The figure shows three views and two pictorial views of one solid part (mm, origin at its lowest corner). Answer the questions. A direction names the side the tool comes from. Coordinates: 2 decimals unless noted, no trailing zeros. Loops run counter-clockwise (first coordinate to the right, second up) from the corner with the lowest first, then second, coordinate; pieces in that order, holes last.
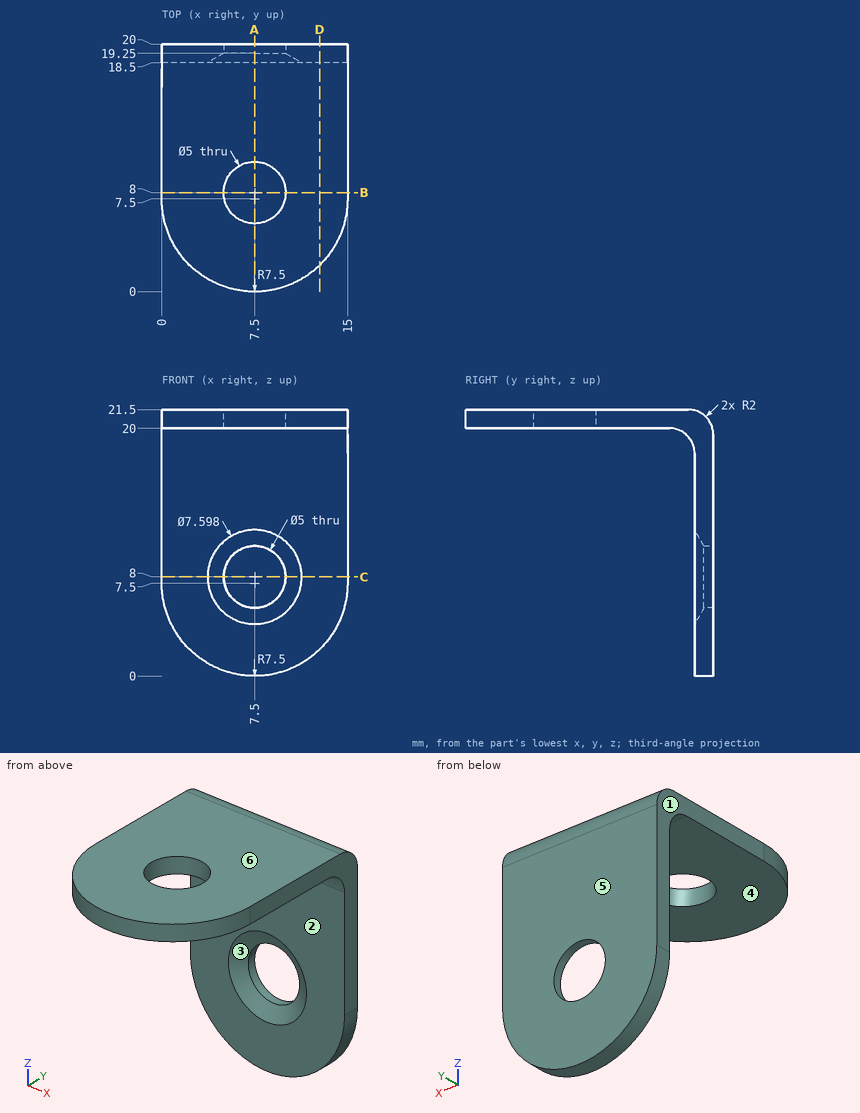
1. Straight lines are drawn through the part: probe 1 along X at (y, z) = (8, 21); probe 2 along Z at (x, y) = (13.5, 15.75); probe 3 along Y at (x, z) = (9, 18). For each, find the intervals that lie inside material, in ascending order.
2. A cutting plane is placed at A-A, the plane x = 7.5. Give the vertices of the cut face in (y, z), then the cut area to 3 significant figures.
3. For the marked faces 1 and 2, determine the directions among +Z, -Z, +X, -X, +Y, -Y from which every point of the face is accessible in a straight line to the end or side of a thin tool.
4. A cutting plane is placed at B-B, the plane y = 8. Give the vertices of the cut face in (x, z).
5. A cutting plane is placed at C-C, the plane z = 8. Give the vertices of the cut face in (x, y).
6. Each of these flat-tipped pins is pushed along its axis until it touches: P1, Ø4, axis at x = 5, z = 16.5, coming from the -Y side; P2, Ø8, axis at x = 7.5, z = 8, coming from the -Y side; P3, Ø4.5, axis at x = 4, y = 4.5, coming from the -Z side; P4, Ø10, axis at y = 17.5, z = 11, coming from the +X side. Where does it stop, or does it pass through?
7. A cutting plane is placed at D-D, the plane x = 12.75. Give the vertices of the cut face in (y, z).
8. Determine the mould class of the marked faces 3, 4, 5 and 6 for opening direction Z: released by +Z, released by -Z, zero draft, split by the parting line, or undercut.
Answers below:
1. probe 1: x = 0 to 5, 10 to 15
1. probe 2: z = 20 to 21.5
1. probe 3: y = 18.5 to 20
2. outline: (0, 20) - (5.5, 20) - (5.5, 21.5) - (0, 21.5) - close; (10.5, 20) - (16.5, 20) arc R2 cw to (18.5, 18) - (18.5, 11.8) - (19.25, 10.5) - (20, 10.5) - (20, 19.5) arc R2 ccw to (18, 21.5) - (10.5, 21.5) - close; (18.5, 0) - (20, 0) - (20, 5.5) - (19.25, 5.5) - (18.5, 4.2) - close
2. area: 44.0 mm2
3. face 1: +Z, -Z, -X, +Y, -Y
3. face 2: -Z, +X, -X, -Y
4. outline: (0, 20) - (5, 20) - (5, 21.5) - (0, 21.5) - close; (10, 20) - (15, 20) - (15, 21.5) - (10, 21.5) - close
5. outline: (0, 18.5) - (3.7, 18.5) - (5, 19.25) - (5, 20) - (0, 20) - close; (10, 19.25) - (11.3, 18.5) - (15, 18.5) - (15, 20) - (10, 20) - close
6. P1: stops at y = 18.44
6. P2: stops at y = 18.5
6. P3: stops at z = 20
6. P4: stops at x = 15
7. outline: (2.14, 20) - (16.5, 20) arc R2 cw to (18.5, 18) - (18.5, 2.14) - (20, 2.14) - (20, 19.5) arc R2 ccw to (18, 21.5) - (2.14, 21.5) - close
8. face 3: undercut
8. face 4: released by -Z
8. face 5: zero draft
8. face 6: released by +Z
